Answer from the drawing. Dimensions are ordinates in mm from the lowest x, y and z of the part. Round coordinates to 2 decimals unless told otherwise and drop trailing zeros. Write each loop counter-clockwise with the first axis right and the second up, starting at its lowest first coordinate (ties: lowest second). Pieces come first, ordered by that corner, then holes. Notation, with made-up numbers: (41, -15.75) -> (80, -15.75) arc R17 ccw to (80, -10.75) -> close; hole circle Ø1 at (11, 44.25). An arc over 180 degrees is marked (long way). Return JSON: item names as keys, results as strings. Group by question number.
(1) Given pin 1 (3.5 mm diameter, centred on y = 2, z = 29.5, fed in from -X); pin 2 (2.5 mm diameter, centred on x = 30.5, y = 2, fed in from +Z); pin 3 (1.8 mm diameter, centred on x = 29.5, z = 11.5, fed in from -Y); pin 4 (1.5 mm diameter, centred on y = 1.5, z = 29.5, fed in from +X), each flat-ended and moving along its own axis, determine where each tip first touches the part or whether it passes through.
(2) The mould has two halves that part along X. Classify the marked faces 1, 2 and 3: released by +X, released by -X, zero draft, split by the parting line, or undercut.
(3) A cutting plane is placed at D-D on x = 9. Give the vertices of the cut face in (y, z).
(4) A cutting plane is placed at B-B on x = 23. Give the vertices of the cut face in (y, z).
(5) A cutting plane is placed at C-C on z = 16.5. Give the vertices of the cut face in (x, y), then the cut area to 3 significant figures.
(6) A cutting plane is placed at A-A on y = 2. Give the vertices of the cut face in (x, z), then the cut area to 3 significant figures.
(7) Straight lines are drawn through the part: line 1 (Z direction, x = 9, y = 1.5); line 2 (X direction, y = 0.5, z = 26); line 3 (X direction, y = 8.5, z = 50). For each, find the intervals that lie inside material, in ascending order.
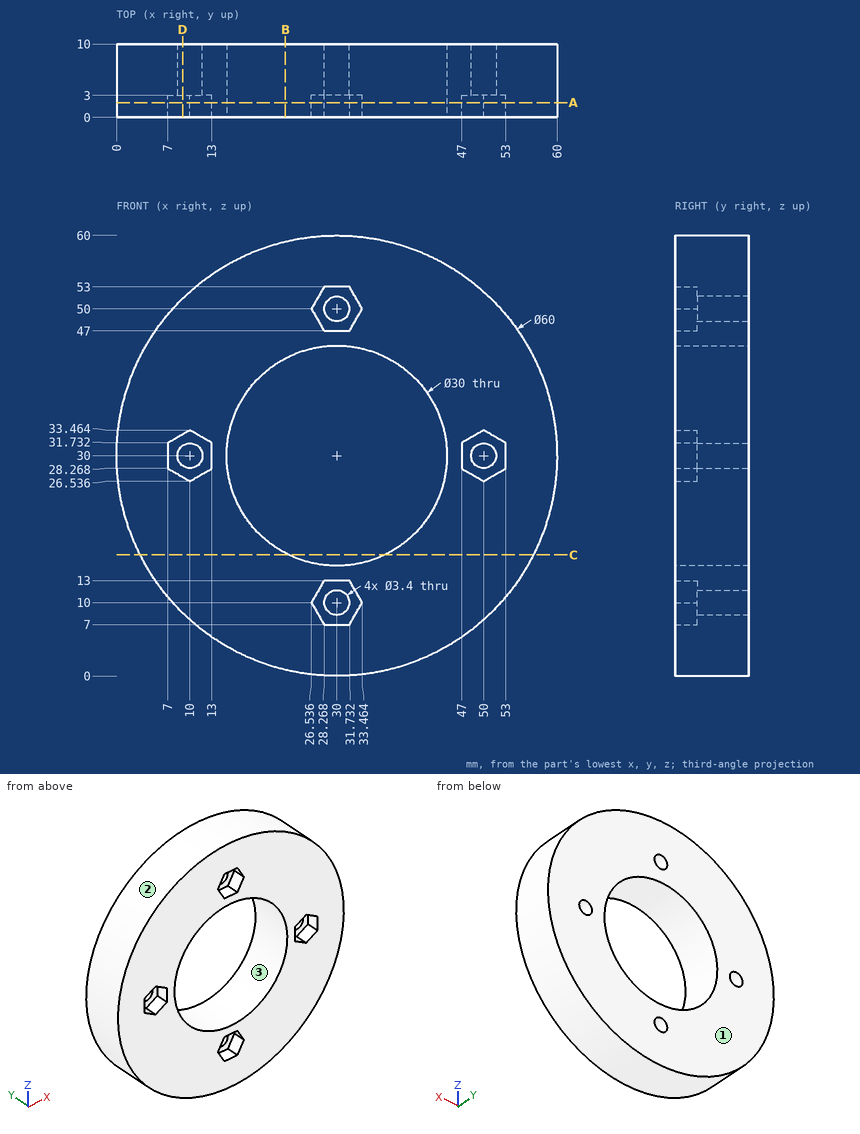
Checks:
{
 "1": {"pin 1": "stops at x = 0", "pin 2": "stops at z = 60", "pin 3": "stops at y = 3", "pin 4": "stops at x = 60"},
 "2": {"face 1": "zero draft", "face 2": "split by the parting line", "face 3": "undercut"},
 "3": {"outline": "(0, 8.58) -> (10, 8.58) -> (10, 28.63) -> (3, 28.63) -> (3, 27.11) -> (0, 27.11) -> close; (0, 32.89) -> (3, 32.89) -> (3, 31.37) -> (10, 31.37) -> (10, 51.42) -> (0, 51.42) -> close"},
 "4": {"outline": "(0, 0.83) -> (10, 0.83) -> (10, 16.73) -> (0, 16.73) -> close; (0, 43.27) -> (10, 43.27) -> (10, 59.17) -> (0, 59.17) -> close"},
 "5": {"outline": "(3.21, 0) -> (23.46, 0) -> (23.46, 10) -> (3.21, 10) -> close; (36.54, 0) -> (56.79, 0) -> (56.79, 10) -> (36.54, 10) -> close", "area": "405 mm^2"},
 "6": {"outline": "circle Ø60 at (30, 30); hole (7, 28.27) -> (10, 26.54) -> (13, 28.27) -> (13, 31.73) -> (10, 33.46) -> (7, 31.73) -> close; hole circle Ø30 at (30, 30); hole (26.54, 10) -> (28.27, 7) -> (31.73, 7) -> (33.46, 10) -> (31.73, 13) -> (28.27, 13) -> close; hole (26.54, 50) -> (28.27, 47) -> (31.73, 47) -> (33.46, 50) -> (31.73, 53) -> (28.27, 53) -> close; hole (47, 28.27) -> (50, 26.54) -> (53, 28.27) -> (53, 31.73) -> (50, 33.46) -> (47, 31.73) -> close", "area": "2,000 mm^2"},
 "7": {"line 1": "z = 8.58 to 27.11, 32.89 to 51.42", "line 2": "x = 0.27 to 15.54, 44.46 to 59.73", "line 3": "x = 7.64 to 28.3, 31.7 to 52.36"}
}
